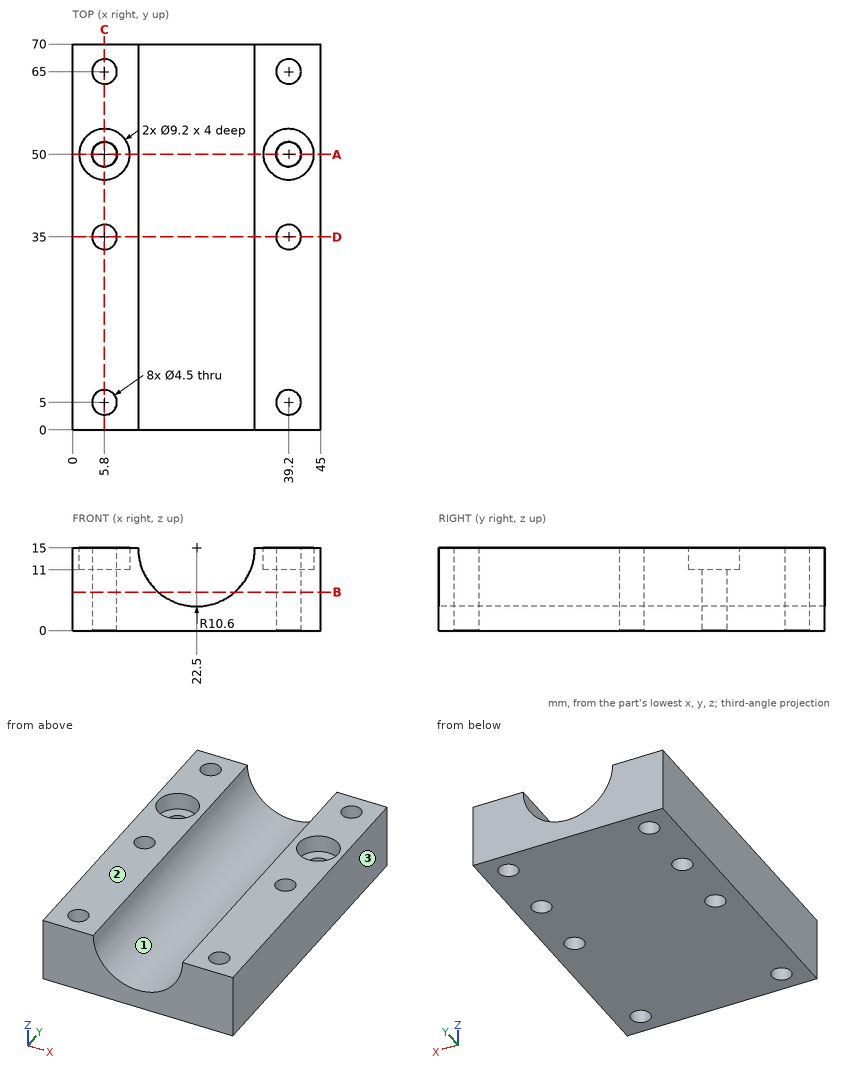
Can you work these out from the drawing? Everything is in mm from the part's minimum corner. Coordinates: 2 decimals unless noted, no trailing zeros. Loops run counter-clockwise (first coordinate to the right, second up) from the corner with the lowest first, then second, coordinate; pieces in that order, holes last. Notation, with made-up numbers: M 74.25,80.25 L 93.25,80.25 A17 cw 93.25,97.25 Z; hole C 50,13 d8. An arc over 180 degrees is marked long. Put each result on its own line as item: value. Start each with the question number.
(1) I need wall thicknesses on line 1 (Y direction, x = 39, z = 6.5); line 2 (X direction, y = 50, z = 2.5); line 3 (X direction, y = 50, z = 5.25). Which ranges of each line are inside material? Lowest first, please. Write a range as from..to.
(2) Suppose I cut it at A-A on y = 50. Please give me the cut outline in (x, z).
(3) Suppose I cut it at B-B on z = 7. Count the separate pieces of the cut face and the enclosed holes in it, then the cut area to 3 significant figures.
(4) Suppose I cut it at C-C on x = 5.8. Please give me the cut outline in (y, z).
(5) Thinking about a two-plate mould opening in X: for the marked faces 1, 2 and 3, which applies, pulls with the +X half, pulls with the -X half, needs draft (parallel to the pull), parting line crosses it, or undercut?
(6) Suppose I cut it at D-D on y = 35. Please give me the cut outline in (x, z), then the cut area to 3 significant figures.
Solutions:
1. line 1: y = 0..2.76, 7.24..32.76, 37.24..47.76, 52.24..62.76, 67.24..70
1. line 2: x = 0..3.55, 8.05..36.95, 41.45..45
1. line 3: x = 0..3.55, 8.05..18.34, 26.66..36.95, 41.45..45
2. outline: M 0,0 L 3.55,0 L 3.55,11 L 1.2,11 L 1.2,15 L 0,15 Z; M 8.05,0 L 36.95,0 L 36.95,11 L 34.6,11 L 34.6,15 L 33.1,15 A10.6 cw 11.9,15 L 10.4,15 L 10.4,11 L 8.05,11 Z; M 41.45,0 L 45,0 L 45,15 L 43.8,15 L 43.8,11 L 41.45,11 Z
3. separate pieces: 2
3. enclosed holes: 8
3. area: 2,050 mm2
4. outline: M 0,0 L 2.75,0 L 2.75,15 L 0,15 Z; M 7.25,0 L 32.75,0 L 32.75,15 L 7.25,15 Z; M 37.25,0 L 47.75,0 L 47.75,11 L 45.4,11 L 45.4,15 L 37.25,15 Z; M 52.25,0 L 62.75,0 L 62.75,15 L 54.6,15 L 54.6,11 L 52.25,11 Z; M 67.25,0 L 70,0 L 70,15 L 67.25,15 Z
5. face 1: undercut
5. face 2: needs draft
5. face 3: pulls with the +X half
6. outline: M 0,0 L 3.55,0 L 3.55,15 L 0,15 Z; M 8.05,0 L 36.95,0 L 36.95,15 L 33.1,15 A10.6 cw 11.9,15 L 8.05,15 Z; M 41.45,0 L 45,0 L 45,15 L 41.45,15 Z
6. area: 364 mm2
